from build123d import *

# Parameters (mm, degrees)
F0_W      = 25.4
F0_H      = 25.4
F1_DEPTH  = 25.4
F7_D      = 2.54
F7_DEPTH  = 1.27
F7_TIP    = 0.7630929862
F8_D      = 2.54
F8_DEPTH  = 1.27
F8_TIP    = 0.7630929862
F9_D      = 2.54
F9_DEPTH  = 1.27
F9_TIP    = 0.7630929862
F10_D     = 2.54
F10_DEPTH = 1.27
F10_TIP   = 0.7630929862
F11_D     = 2.54
F11_DEPTH = 1.27
F11_TIP   = 0.7630929862
F12_D     = 2.54
F12_DEPTH = 1.27
F12_TIP   = 0.7630929862


with BuildPart() as f1:
    # F0 (on Top) → F1 (new body)
    with BuildSketch(Plane.XY):
        Rectangle(F0_W, F0_H)
    extrude(amount=F1_DEPTH)

    # F7
    with Locations(Plane.XY.offset(25.4)):
        with Locations((-6.35, 6.35), (6.35, 6.35), (-6.35, 0), (-6.35, -6.35), (6.35, 0), (6.35, -6.35)):
            Hole(F7_D / 2, depth=F7_DEPTH)
            with Locations((0, 0, -(F7_DEPTH + F7_TIP / 2))):  # 118° drill point
                Cone(0, F7_D / 2, F7_TIP, mode=Mode.SUBTRACT)

    # F8
    with Locations(Plane.XZ.offset(12.7)):
        with Locations((-6.35, 19.05), (6.35, 19.05), (6.35, 6.35), (-6.35, 6.35)):
            Hole(F8_D / 2, depth=F8_DEPTH)
            with Locations((0, 0, -(F8_DEPTH + F8_TIP / 2))):  # 118° drill point
                Cone(0, F8_D / 2, F8_TIP, mode=Mode.SUBTRACT)

    # F9
    with Locations(Plane(origin=(-12.7, 0, 0), x_dir=(0, -1, 0), z_dir=(-1, 0, 0))):
        with Locations((-6.35, 6.35), (-6.35, 19.05), (6.35, 19.05), (6.35, 6.35), (0, 12.7)):
            Hole(F9_D / 2, depth=F9_DEPTH)
            with Locations((0, 0, -(F9_DEPTH + F9_TIP / 2))):  # 118° drill point
                Cone(0, F9_D / 2, F9_TIP, mode=Mode.SUBTRACT)

    # F10
    with Locations(Plane(origin=(0, 12.7, 0), x_dir=(-1, 0, 0), z_dir=(0, 1, 0))):
        with Locations((6.35, 6.35), (0, 12.7), (-6.35, 19.05)):
            Hole(F10_D / 2, depth=F10_DEPTH)
            with Locations((0, 0, -(F10_DEPTH + F10_TIP / 2))):  # 118° drill point
                Cone(0, F10_D / 2, F10_TIP, mode=Mode.SUBTRACT)

    # F11
    with Locations(Plane(origin=(0, 0, 0), x_dir=(1, 0, 0), z_dir=(0, 0, -1))):
        with Locations((0, 0)):
            Hole(F11_D / 2, depth=F11_DEPTH)
            with Locations((0, 0, -(F11_DEPTH + F11_TIP / 2))):  # 118° drill point
                Cone(0, F11_D / 2, F11_TIP, mode=Mode.SUBTRACT)

    # F12
    with Locations(Plane.YZ.offset(12.7)):
        with Locations((-6.35, 19.05), (6.35, 6.35)):
            Hole(F12_D / 2, depth=F12_DEPTH)
            with Locations((0, 0, -(F12_DEPTH + F12_TIP / 2))):  # 118° drill point
                Cone(0, F12_D / 2, F12_TIP, mode=Mode.SUBTRACT)


solid = f1.part
Can you work these out from the model? Positions are in its coordinate system, mm. A direction names the side the tool comes from. Round coordinates to 2 decimals unless told otherwise and drop trailing zeros. Answer in a Markdown table with one row per item. Add a question column.
Q1. Which directions (+Z, -Z, +X, -X, +Y, -Y) give clear straight access to the entire face, cutting with the end or side of a thin tool? Please do faces 5 (the cylindrical face through (6.18, 12.06, 20.31)), 6 (the cylindrical face through (7.62, 0.06, 24.76)), 7 (the cylindrical face through (-12.06, -0.17, 13.96)), 8 (the cylindrical face through (-6.18, -12.06, 20.31)).
Q2. We'd pull the mould along X, two halves only. Please class faces 1 (the conical face through (6.19, 6.5, 23.5)), 2 (the conical face through (10.799, -6.398, 18.835)), 3 (the cylindrical face through (-12.06, 6.18, 20.31)), 4 (the cylindrical face through (-6.07, -7.59, 24.76)): pulls with the +X half, pulls with the -X half, needs draft (parallel to the pull), parting line crosses it, or undercut.
Q3. For pin 1 Ø1.5 at (x, y) = (0, 0) entering from -Z; pin 2 Ø1.5 at (x, z) = (-6.35, 6.35) entering from +Y; pin 3 Ø2 at (x, z) = (-6.35, 19.05) entering from -Y, each with a flat end and sliding along its axis, tell me the tip position at first contact or that it passes through.
Q4. I need wall thicknesses on L1, parallel to Z at x = -12.25, y = 6.35; L2, parallel to X at y = 0, z = 24.75; L3, parallel to Y at x = -6.35, z = 24.65. Which ranges of each line are inside material? Lowest first, please.
A:
| question | item | result |
|---|---|---|
| 1 | face 5 | +Y |
| 1 | face 6 | +Z |
| 1 | face 7 | -X |
| 1 | face 8 | -Y |
| 2 | face 1 | undercut |
| 2 | face 2 | pulls with the +X half |
| 2 | face 3 | needs draft |
| 2 | face 4 | undercut |
| 3 | pin 1 | z = 1.58 |
| 3 | pin 2 | y = 11.12 |
| 3 | pin 3 | y = -11.27 |
| 4 | L1 | 0 to 5.08, 7.62 to 17.78, 20.32 to 25.4 |
| 4 | L2 | -12.7 to -7.62, -5.08 to 5.08, 7.62 to 12.7 |
| 4 | L3 | -12.7 to -7.62, -5.08 to -1.27, 1.27 to 5.08, 7.62 to 12.7 |
